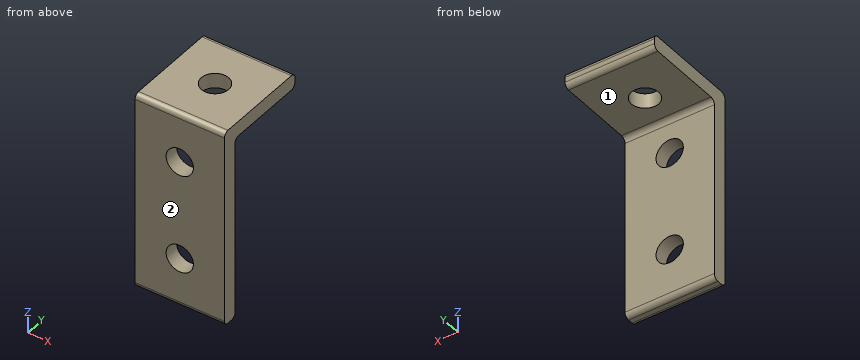
```python
from build123d import *

# Parameters (mm, degrees)
SKETCH_1_W          = 40
SKETCH_1_H          = 20
EXTRUDE_1_DEPTH     = 18
SKETCH_2_W          = 37
SKETCH_2_H          = 17
CUT_EXTRUDE_1_DEPTH = 18
SKETCH_3_R          = 2.75
CUT_EXTRUDE_2_DEPTH = 18
SKETCH_4_R          = 2.75
CUT_EXTRUDE_3_DEPTH = 18
FILLET_1_R          = 1


with BuildPart() as part:
    # 草图1 → 凸台-拉伸1 (new body)
    with BuildSketch(Plane(origin=(0, 0, 0), x_dir=(0, 0, -1), z_dir=(1, 0, 0))):
        with Locations((20, 10)):
            Rectangle(SKETCH_1_W, SKETCH_1_H)
    extrude(amount=EXTRUDE_1_DEPTH)

    # 草图2 → 切除-拉伸1 (cut)
    with BuildSketch(Plane(origin=(18, 0, 0), x_dir=(0, 0, -1), z_dir=(1, 0, 0))):
        with Locations((21.5, 11.5)):
            Rectangle(SKETCH_2_W, SKETCH_2_H)
    extrude(amount=-CUT_EXTRUDE_1_DEPTH, mode=Mode.SUBTRACT)

    # 草图3 → 切除-拉伸2 (cut)
    with BuildSketch(Plane(origin=(0, 0, -3), x_dir=(-1, 0, 0), z_dir=(0, 0, -1))):
        with Locations((-9, 10)):
            Circle(SKETCH_3_R)
    extrude(amount=-CUT_EXTRUDE_2_DEPTH, mode=Mode.SUBTRACT)

    # 草图4 → 切除-拉伸3 (cut)
    with BuildSketch(Plane(origin=(0, 3, 0), x_dir=(1, 0, 0), z_dir=(0, 1, 0))):
        with Locations(Location((9, 30, 0), (0, 0, 270))):
            Circle(SKETCH_4_R)
        with Locations(Location((9, 10, 0), (0, 0, 270))):
            Circle(SKETCH_4_R)
    extrude(amount=-CUT_EXTRUDE_3_DEPTH, mode=Mode.SUBTRACT)

    # 圆角1
    fillet_1_edges = [part.edges().sort_by_distance(p)[0] for p in [
        (9, 20, -3),
        (9, 3, -40),
        (9, 3, -3),
        (9, 20, 0),
        (9, 0, -40),
        (9, 0, 0),
    ]]
    fillet(fillet_1_edges, radius=FILLET_1_R)


solid = part.part
```
Here's how the part is built. I have some questions about the finished solid (model axes, mm). Face numbers are marked on the shaded views. A direction names the side the tool comes from. Coordinates: 2 decimals unless noted, no trailing zeros. Write each loop counter-clockwise with the first axis right and the second up, starting at its lowest first coordinate (ties: lowest second). Pieces come first, ordered by that corner, then holes. Notation, with made-up numbers: (17.5, 59.5) - (26.5, 59.5) arc R31 cw to (26.5, 97.5) - close; hole circle Ø2 at (-5.75, 56.5). An arc over 180 degrees is marked (long way). One line per item, written item: value.
1) I'm going to push flat-ended pins straight in: P1, Ø6.5, axis at x = 9, z = -30, coming from the +Y side; P2, Ø6.5, axis at x = 9, y = 10, coming from the +Z side; P3, Ø1.5, axis at x = 10, y = 17, coming from the -Z side. Where does each tip first touch, or does it pass through?
Model answer:
P1: stops at y = 3
P2: stops at z = 0
P3: stops at z = -3
2) Suppose I cut it at C-C on x = 9. Write out the boundary of the cut face in (y, z), and give its area (3 significant figures).
Model answer:
outline: (0, -39) arc R1 ccw to (1, -40) - (2, -40) arc R1 ccw to (3, -39) - (3, -32.75) - (0, -32.75) - close; (0, -27.25) - (3, -27.25) - (3, -12.75) - (0, -12.75) - close; (0, -7.25) - (3, -7.25) - (3, -4) arc R1 cw to (4, -3) - (7.25, -3) - (7.25, 0) - (1, 0) arc R1 ccw to (0, -1) - close; (12.75, -3) - (19, -3) arc R1 ccw to (20, -2) - (20, -1) arc R1 ccw to (19, 0) - (12.75, 0) - close
area: 121 mm²
3) Suppose I cut it at B-B on z = -30. Write out the boundary of the cut face in (x, y), and give its area (3 significant figures).
Model answer:
outline: (0, 0) - (6.25, 0) - (6.25, 3) - (0, 3) - close; (11.75, 0) - (18, 0) - (18, 3) - (11.75, 3) - close
area: 37.5 mm²
4) Suppose I cut it at A-A on y = 10. Write out the boundary of the cut face in (x, z).
Model answer:
outline: (0, -3) - (6.25, -3) - (6.25, 0) - (0, 0) - close; (11.75, -3) - (18, -3) - (18, 0) - (11.75, 0) - close
5) Suppose I cut it at D-D on x = 12.75. Write out the boundary of the cut face in (y, z).
Model answer:
outline: (0, -39) arc R1 ccw to (1, -40) - (2, -40) arc R1 ccw to (3, -39) - (3, -4) arc R1 cw to (4, -3) - (19, -3) arc R1 ccw to (20, -2) - (20, -1) arc R1 ccw to (19, 0) - (1, 0) arc R1 ccw to (0, -1) - close
6) I need wall thicknesses on line 1 along X through (y, z) = (2.15, -30); line 2 along Y through (x, z) = (9, -2); line 3 along Y through (x, z) = (9.5, -26.5). Which ranges of each line are inside material? Lowest first, please.
Model answer:
line 1: x = 0 to 6.25, 11.75 to 18
line 2: y = 0 to 7.25, 12.75 to 20
line 3: y = 0 to 3
7) On a 3-axis mill with a long thin cutter (end or side, diameter ignored), from which of +Z, -Z, +X, -X, +Y, -Y can I reach the whole of each face in a straight line? I mean the marked faces 1 and 2. Say none if no direction works.
Model answer:
face 1: -Z, +X, -X, +Y
face 2: +Z, -Z, +X, -X, -Y
